Part model, mm, in its own coordinate system. Face numbers are marked on the shaded views. A direction names the side the tool comes from. Coordinates: 2 decimals unless noted, no trailing zeros. Order: outer loops, then holes, each group sorted by start corner. A loop starts at its lowest first (then second) coordinate and runs counter-clockwise, first axis right, second up.
1) Cut at A-A (y = -6.75). List the corners of the cut face in (x, z), and give its area (3 significant figures).
2) Cut at D-D (z = 5). List the corners of the cut face in (x, y).
3) Cut at B-B (y = -2.25). List the corners of the cut face in (x, z).
4) Wall check: L1, parallel to Z at x = -5, y = 5; L2, parallel to Z at x = -26, y = 5.5; L3, parallel to X at y = -6, z = 13. Give the ranges that are in metal, low to high.
5) Cut at C-C (x = -2). List the corners of the cut face in (y, z).
6) Pin check, flat tips, straight feed: pin 1 Ø5 at (x, y) = (28.5, 1) entering from +Z; pin 2 Ø2 at (x, z) = (-5.5, 8) entering from +Y; pin 3 Ø5 at (x, z) = (-1.5, 7.5) entering from -Y; pin 4 Ø3 at (x, z) = (-13.5, 5) entering from -Y. Stop position of each tip, or through.
7) Mould opens along Z. For the marked faces 4, 5, 6 and 7 say: +Z half, -Z half, draft (parallel to the pull), parting line (faces both ways), or undercut.
8) Tool access for the marked faces 1, 2 and 3: list every direction of +Z, -Z, +X, -X, +Y, -Y with a clear straight run to the whole face (end or side of a thin tool).
```python
from build123d import *

# Parameters (mm, degrees)
SKETCH1_W           = 78
SKETCH1_H           = 16
BOSS_EXTRUDE1_DEPTH = 2
SKETCH2_W           = 13
SKETCH2_H           = 8
BOSS_EXTRUDE2_DEPTH = 9.5
SKETCH3_W           = 13
SKETCH3_H           = 24
BOSS_EXTRUDE3_DEPTH = 3


with BuildPart() as part:
    # Sketch1 → Boss-Extrude1 (new body)
    with BuildSketch(Plane.XY):
        Rectangle(SKETCH1_W, SKETCH1_H)
    extrude(amount=BOSS_EXTRUDE1_DEPTH)

    # Sketch2 → Boss-Extrude2 (add)
    with BuildSketch(Plane.XY.offset(2)):
        Rectangle(SKETCH2_W, SKETCH2_H)
    extrude(amount=BOSS_EXTRUDE2_DEPTH)

    # Sketch3 → Boss-Extrude3 (add)
    with BuildSketch(Plane.XY.offset(11.5)):
        Rectangle(SKETCH3_W, SKETCH3_H)
    extrude(amount=BOSS_EXTRUDE3_DEPTH)


solid = part.part
```
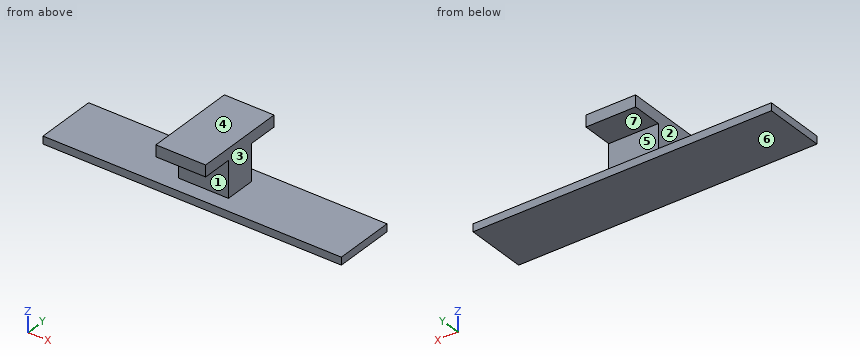
Geometry check:
1. outline: (-39, 0) - (39, 0) - (39, 2) - (-39, 2) - close; (-6.5, 11.5) - (6.5, 11.5) - (6.5, 14.5) - (-6.5, 14.5) - close
1. area: 195 mm2
2. outline: (-6.5, -4) - (6.5, -4) - (6.5, 4) - (-6.5, 4) - close
3. outline: (-39, 0) - (39, 0) - (39, 2) - (6.5, 2) - (6.5, 14.5) - (-6.5, 14.5) - (-6.5, 2) - (-39, 2) - close
4. L1: z = 0 to 2, 11.5 to 14.5
4. L2: z = 0 to 2
4. L3: x = -6.5 to 6.5
5. outline: (-12, 11.5) - (-4, 11.5) - (-4, 2) - (-8, 2) - (-8, 0) - (8, 0) - (8, 2) - (4, 2) - (4, 11.5) - (12, 11.5) - (12, 14.5) - (-12, 14.5) - close
6. pin 1: stops at z = 2
6. pin 2: stops at y = 4
6. pin 3: stops at y = -4
6. pin 4: passes through
7. face 4: +Z half
7. face 5: undercut
7. face 6: -Z half
7. face 7: undercut
8. face 1: +X, -X, -Y
8. face 2: +Z, -X, +Y, -Y
8. face 3: +Z, +X, +Y, -Y
